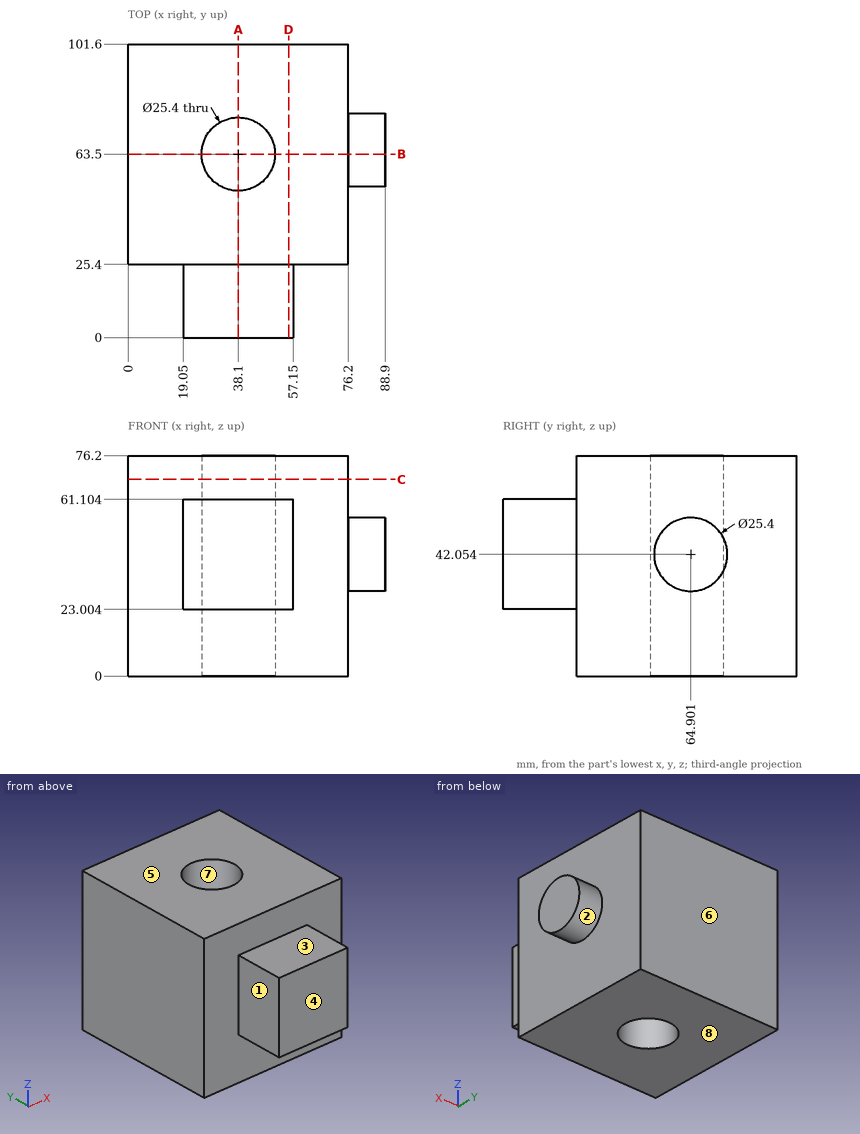
Geometry check sheet. Reference: drawing and pictorial views, mm from the part's lowest x, y, z. A direction names the side the tool comes from. Round coordinates to 2 decimals unless told otherwise and drop trailing zeros. Write each loop counter-clockwise with the first axis right and the second up, starting at its lowest first coordinate (ties: lowest second). Pieces come first, ordered by that corner, then holes.
(1) Section check B-B (y = 63.5). Enter the section's corners in (x, z), plus the area to 3 significant figures.
Returned:
outline: (0, 0) - (25.4, 0) - (25.4, 76.2) - (0, 76.2) - close; (50.8, 0) - (76.2, 0) - (76.2, 29.43) - (88.9, 29.43) - (88.9, 54.68) - (76.2, 54.68) - (76.2, 76.2) - (50.8, 76.2) - close
area: 4,190 mm2
(2) Depth check by flat-ended pin: pin 1 Ø12.5 at (x, y) = (44.5, 7) entering from -Z; pin 2 Ø5 at (y, z) = (43.5, 59.5) entering from +X; pin 3 Ø4 at (x, y) = (48.5, 62.5) entering from +Z; pin 4 Ø12.5 at (x, y) = (39, 12.5) entering from +Z. Enter the tip coordinate at first touch or a pass-through.
Returned:
pin 1: stops at z = 23
pin 2: stops at x = 76.2
pin 3: passes through
pin 4: stops at z = 61.1
(3) Section check A-A (x = 38.1). Enter the section's corners in (y, z), plus the area to 3 significant figures.
Returned:
outline: (0, 23) - (25.4, 23) - (25.4, 0) - (50.8, 0) - (50.8, 76.2) - (25.4, 76.2) - (25.4, 61.1) - (0, 61.1) - close; (76.2, 0) - (101.6, 0) - (101.6, 76.2) - (76.2, 76.2) - close
area: 4,840 mm2
(4) Section check C-C (z = 68). Enter the section's corners in (x, y), plus the area to 3 significant figures.
Returned:
outline: (0, 25.4) - (76.2, 25.4) - (76.2, 101.6) - (0, 101.6) - close; hole circle Ø25.4 at (38.1, 63.5)
area: 5,300 mm2
(5) Material ranges on line 1 (Y direction, x = 38.1, z = 21); line 2 (Y direction, x = 38.1, z = 35); line 3 (Y direction, x = 20.5, z = 72.5), recorded low to high.
Returned:
line 1: y = 25.4 to 50.8, 76.2 to 101.6
line 2: y = 0 to 50.8, 76.2 to 101.6
line 3: y = 25.4 to 101.6
(6) Section check D-D (x = 55.5). Enter the section's corners in (y, z), plus the area to 3 significant figures.
Returned:
outline: (0, 23) - (25.4, 23) - (25.4, 0) - (101.6, 0) - (101.6, 76.2) - (25.4, 76.2) - (25.4, 61.1) - (0, 61.1) - close
area: 6,770 mm2
(7) Mould release check, pull along Y, two halves, no side actions. Record for the marked faces 6, 7 and 8: pulls with the +Y half, pulls with the -Y half, needs draft (parallel to the pull), parting line crosses it, or undercut.
Returned:
face 6: pulls with the +Y half
face 7: undercut
face 8: needs draft
(8) Access from +Z, -Z, +X, -X, +Y, -Y to the whole of each face (thin tool, end or side, straight path). Record for the marked faces 1, 2, 3, 4 and 5.
Returned:
face 1: +Z, -Z, -X, -Y
face 2: +X
face 3: +Z, +X, -X, -Y
face 4: +Z, -Z, +X, -X, -Y
face 5: +Z, +X, -X, +Y, -Y
